Verification items for the finished model (mm, model axes). Round coordinates to 2 decimals unless told otherwise and drop trailing zeros. Order: outer loops, then holes, each group sorted by start corner. A loop starts at its lowest first (then second) coordinate and runs counter-clockwise, first axis right, second up. Notation, with made-up numbers: (30, 18.5) -> (69, 18.5) arc R26 cw to (69, 37.5) -> close; hole circle Ø10 at (-17.75, 25.25). An arc over 180 degrees is marked (long way). Return JSON: item names as keys, results as strings. Group by question number.
1) Section check C-C on x = 67. Enter the section's corners in (y, z), plus the area to 3 significant figures.
2) Depth check by flat-ended pin: pin 1 (0.6 mm diameter, centred on y = 5.5, z = -1, fed in from +X); pin 2 (3.5 mm diameter, centred on x = 84.9, y = 84.9, fed in from -Z); pin 3 (1 mm diameter, centred on x = 122.5, z = -0.5, fed in from +Y); pin 4 (0.6 mm diameter, centred on x = 6, z = -1, fed in from +Y). Enter the tip coordinate at first touch or a pass-through.
3) Section check A-A on y = 84.9. Enter the section's corners in (x, z).
4) Scan lines: L1, parallel to X at y = 6.5, z = -1.25; L2, parallel to Y at x = 84.9, z = -0.85; L3, parallel to X at y = 17.5, z = -0.8. Record each from-to range of solid material in increasing order.
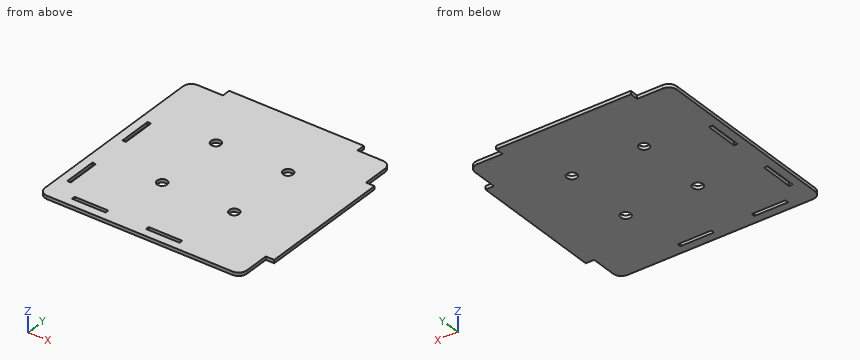
```python
from build123d import *

# Parameters (mm, degrees)
SKETCH1_R          = 3
SKETCH1_W          = 20
SKETCH1_H          = 2.1
SKETCH1_W_2        = 2.1
SKETCH1_H_2        = 20
BASE_FLANGE1_DEPTH = 2
FILLET1_R          = 5


# Sheet-metal steps are written as plain solids
with BuildPart() as part:
    # Sketch1 → Base-Flange1 (new body)
    with BuildSketch(Plane.XY):
        Polygon((0, 0), (120, 0), (120, 20), (125, 20), (125, 100), (120, 100), (120, 120), (100, 120), (100, 125), (20, 125), (20, 120), (0, 120), align=None)
        with Locations((42, 42)):
            Circle(SKETCH1_R, mode=Mode.SUBTRACT)
        with Locations((84.9, 42)):
            Circle(SKETCH1_R, mode=Mode.SUBTRACT)
        with Locations((42, 84.9)):
            Circle(SKETCH1_R, mode=Mode.SUBTRACT)
        with Locations((84.9, 84.9)):
            Circle(SKETCH1_R, mode=Mode.SUBTRACT)
        with Locations((26, 6.05)):
            Rectangle(SKETCH1_W, SKETCH1_H, mode=Mode.SUBTRACT)
        with Locations((70, 6.05)):
            Rectangle(SKETCH1_W, SKETCH1_H, mode=Mode.SUBTRACT)
        with Locations((6.05, 26)):
            Rectangle(SKETCH1_W_2, SKETCH1_H_2, mode=Mode.SUBTRACT)
        with Locations((6.05, 70)):
            Rectangle(SKETCH1_W_2, SKETCH1_H_2, mode=Mode.SUBTRACT)
    extrude(amount=-BASE_FLANGE1_DEPTH)

    # Fillet1
    fillet1_edges = [part.edges().sort_by_distance(p)[0] for p in [
        (0, 120, -1),
        (120, 120, -1),
        (120, 0, -1),
        (0, 0, -1),
    ]]
    fillet(fillet1_edges, radius=FILLET1_R)


solid = part.part
```
Check result:
{
 "1": {"outline": "(0, -2) -> (5, -2) -> (5, 0) -> (0, 0) -> close; (7.1, -2) -> (125, -2) -> (125, 0) -> (7.1, 0) -> close", "area": "246 mm^2"},
 "2": {"pin 1": "x = 120", "pin 2": "through", "pin 3": "y = 100", "pin 4": "y = 120"},
 "3": {"outline": "(0, -2) -> (39, -2) -> (39, 0) -> (0, 0) -> close; (45, -2) -> (81.9, -2) -> (81.9, 0) -> (45, 0) -> close; (87.9, -2) -> (125, -2) -> (125, 0) -> (87.9, 0) -> close"},
 "4": {"L1": "0 to 16, 36 to 60, 80 to 120", "L2": "0 to 39, 45 to 81.9, 87.9 to 125", "L3": "0 to 5, 7.1 to 120"}
}
